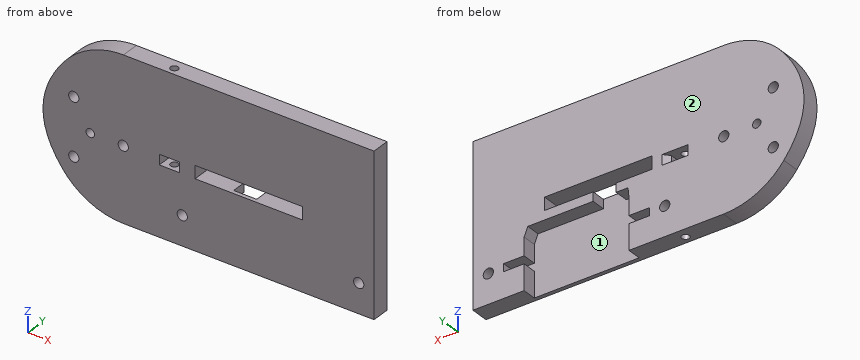
from build123d import *

# Parameters (mm, degrees)
BOSS_EXTRU_1_DEPTH      = 7
ENL_V_MAT_EXTRU_1_DEPTH = 5.5
ESQUISSE3_W             = 42
ESQUISSE3_H             = 5
ENL_V_MAT_EXTRU_2_DEPTH = 7
ESQUISSE4_R             = 2
ENL_V_MAT_EXTRU_3_DEPTH = 7
ESQUISSE5_W             = 8
ESQUISSE5_H             = 4
ENL_V_MAT_EXTRU_4_DEPTH = 7
CHANFREIN1_SIZE         = 2
CHANFREIN1_SIZE2        = 2.22122503
ESQUISSE6_R             = 2
ESQUISSE6_R_2           = 1.65
ENL_V_MAT_EXTRU_5_DEPTH = 7
ESQUISSE7_R             = 1.5
ENL_V_MAT_EXTRU_6_DEPTH = 67
CONG_1_R                = 30


with BuildPart() as part:
    # Esquisse1 → Boss.-Extru.1 (new body)
    with BuildSketch(Plane(origin=(0, 0, 0), x_dir=(1, 0, 0), z_dir=(0, 1, 0))):
        with BuildLine():
            Line((0, 0), (110, 0))
            Line((110, 0), (110, 63))
            Line((110, 63), (0, 63))
            add(Edge.make_bspline(
                [(0, 63), (-38.954434005, 31.5), (0, 0)],
                knots=[0, 0, 0, 1, 1, 1], degree=2))
        make_face()
    extrude(amount=BOSS_EXTRU_1_DEPTH)

    # Esquisse2 → Enlèv. mat.-Extru.1 (cut)
    with BuildSketch(Plane(origin=(0, 7, 0), x_dir=(1, 0, 0), z_dir=(0, 1, 0))):
        Polygon((90, 63), (90, 53), (98, 53), (98, 50), (90, 50), (90, 43), (88.548308046, 39.540825664), (63, 39.540825664), (63, 35.886046781), (54, 35.886046781), (54, 39.466527525), (49.383125702, 39.466527525), (49, 43), (49, 50), (41, 50), (41, 53), (49, 53), (49, 63), align=None)
    extrude(amount=-ENL_V_MAT_EXTRU_1_DEPTH, mode=Mode.SUBTRACT)

    # Esquisse3 → Enlèv. mat.-Extru.2 (cut)
    with BuildSketch(Plane(origin=(0, 7, 0), x_dir=(1, 0, 0), z_dir=(0, 1, 0))):
        with Locations((61, 33.5)):
            Rectangle(ESQUISSE3_W, ESQUISSE3_H)
    extrude(amount=-ENL_V_MAT_EXTRU_2_DEPTH, mode=Mode.SUBTRACT)

    # Esquisse4 → Enlèv. mat.-Extru.3 (cut)
    with BuildSketch(Plane(origin=(0, 7, 0), x_dir=(1, 0, 0), z_dir=(0, 1, 0))):
        with Locations(Location((104, 51.5, 0), (0, 0, 270))):
            Circle(ESQUISSE4_R)
        with Locations(Location((35, 51.5, 0), (0, 0, 270))):
            Circle(ESQUISSE4_R)
    extrude(amount=-ENL_V_MAT_EXTRU_3_DEPTH, mode=Mode.SUBTRACT)

    # Esquisse5 → Enlèv. mat.-Extru.4 (cut)
    with BuildSketch(Plane(origin=(0, 7, 0), x_dir=(1, 0, 0), z_dir=(0, 1, 0))):
        with Locations((30, 33.95274738)):
            Rectangle(ESQUISSE5_W, ESQUISSE5_H)
    extrude(amount=-ENL_V_MAT_EXTRU_4_DEPTH, mode=Mode.SUBTRACT)

    # Chanfrein1
    chanfrein1_edges = [part.edges().sort_by_distance(p)[0] for p in [
        (34, 7, -33.95274738),
    ]]
    chanfrein1_side = [part.faces().sort_by_distance(p)[0] for p in [
        (44.621272822, 7, -28.216818426),
    ]]
    chamfer(chanfrein1_edges, length=CHANFREIN1_SIZE, length2=CHANFREIN1_SIZE2, reference=chanfrein1_side[0])

    # Esquisse6 → Enlèv. mat.-Extru.5 (cut)
    with BuildSketch(Plane(origin=(0, 7, 0), x_dir=(1, 0, 0), z_dir=(0, 1, 0))):
        with Locations(Location((11.916860307, 33.95274738, 0), (0, 0, 270))):
            Circle(ESQUISSE6_R)
        with Locations(Location((-7.438807468, 45.12774738, 0), (0, 0, 270))):
            Circle(ESQUISSE6_R)
        with Locations(Location((-7.438807468, 22.77774738, 0), (0, 0, 270))):
            Circle(ESQUISSE6_R)
        with Locations(Location((-0.986918209, 33.95274738, 0), (0, 0, 270))):
            Circle(ESQUISSE6_R_2)
    extrude(amount=-ENL_V_MAT_EXTRU_5_DEPTH, mode=Mode.SUBTRACT)

    # Esquisse7 → Enlèv. mat.-Extru.6 (cut)
    with BuildSketch(Plane(origin=(0, 0, -63), x_dir=(-1, 0, 0), z_dir=(0, 0, -1))):
        with Locations((-29.749983128, 3)):
            Circle(ESQUISSE7_R)
    extrude(amount=-ENL_V_MAT_EXTRU_6_DEPTH, mode=Mode.SUBTRACT)

    # Congé1
    cong_1_edges = [part.edges().sort_by_distance(p)[0] for p in [
        (0, 3.5, 0),
        (0, 3.5, -63),
    ]]
    fillet(cong_1_edges, radius=CONG_1_R)


solid = part.part
For this review, take the finished solid that the model builds, in its own axes (mm). Face numbers are marked on the shaded views. Round coordinates to 2 decimals unless told otherwise and drop trailing zeros. Loops run counter-clockwise (first coordinate to the right, second up) from the corner with the lowest first, then second, coordinate; pieces in that order, holes last. Notation, with made-up numbers: (70.5, -7) - (115.5, -7) arc R24 ccw to (115.5, 29) - close; hole circle Ø9 at (78.5, 39). An arc over 180 degrees is marked (long way). Put each result on its own line as item: value. Start each with the question number.
1. For probe 1 along X at (y, z) = (2.75, -51.5); probe 2 along Z at (x, y) = (30.5, 1.25); probe 3 along X at (y, z) = (1, -34.5), list the stretches that pass through material, from the lowest coordinate up. Write a range as [from, to].
2. Consider section B-B on y = 3. State how many separate pieces and enclosed holes the cut face has, plus the area to 3 significant figures.
3. Mouldability with a two-part tool opening along X and no side actions: class the marked faces 1 and 2 as +X half, -X half, draft (parallel to the pull), parting line (faces both ways), or undercut.
4. Consider section A-A on x = 104. State the section outline as (y, z) points, plus the area to 3 significant figures.
5. Insertion check: P1, Ø1.8, axis at x = 29.75, y = 3, coming from the +Z side; P2, Ø1, axis at x = 12, y = 4, coming from the +Z side; P3, Ø3.5, axis at x = 69, y = 4, coming from the -Z side; P4, Ø3, axis at x = 88, y = 6, coming from the -Z side. Each pin has a flat end and moves straight along its axis. Give the tip position at first contact, or say it passes through.
Result sheet:
1. probe 1: [-11.63, 28.27], [31.23, 33], [37, 41], [98, 102], [106, 110]
1. probe 2: [-63, -35.95], [-31.95, 0]
1. probe 3: [-19.3, -2.54], [0.57, 9.99], [13.84, 26], [34, 40], [82, 110]
2. separate pieces: 2
2. enclosed holes: 6
2. area: 6,180 mm^2
3. face 1: undercut
3. face 2: draft
4. outline: (0, -63) - (7, -63) - (7, -53.5) - (0, -53.5) - close; (0, -49.5) - (7, -49.5) - (7, 0) - (0, 0) - close
4. area: 413 mm^2
5. P1: through
5. P2: z = 0
5. P3: z = -39.54
5. P4: z = -41.81
